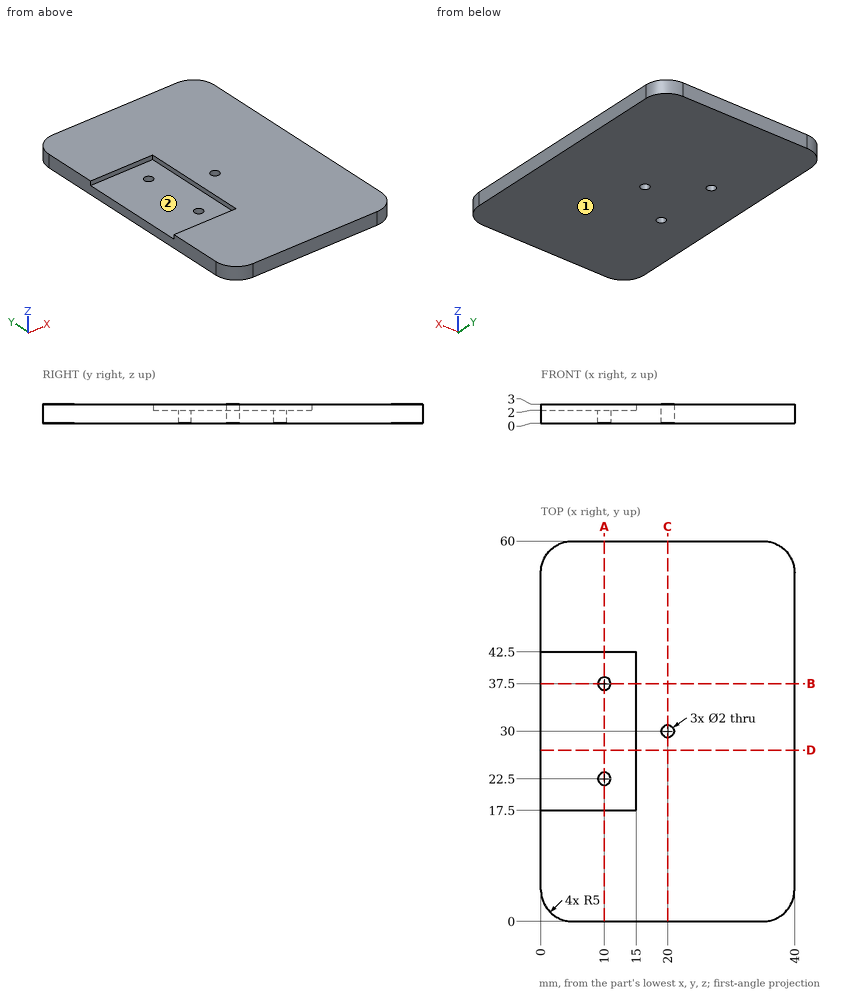
Part print with two shaded views. Sizes in mm from the minimum x, y, z corner. Coordinates: 2 decimals unless noted, no trailing zeros. Order: outer loops, then holes, each group sorted by start corner. A loop starts at its lowest first (then second) coordinate and runs counter-clockwise, first axis right, second up.
(1) Saw through at A-A, the plane x = 10. Write the cut outline in (y, z), and give its area (3 significant figures).
Solution:
outline: (0, 0) - (21.5, 0) - (21.5, 2) - (17.5, 2) - (17.5, 3) - (0, 3) - close; (23.5, 0) - (36.5, 0) - (36.5, 2) - (23.5, 2) - close; (38.5, 0) - (60, 0) - (60, 3) - (42.5, 3) - (42.5, 2) - (38.5, 2) - close
area: 147 mm2
(2) Pin check, flat tips, straight feed: pin 1 Ø2.5 at (x, y) = (10, 37.5) entering from +Z; pin 2 Ø0.5 at (y, z) = (34, 2.5) entering from -X. Stop position of each tip, or through.
Solution:
pin 1: stops at z = 2
pin 2: stops at x = 15
(3) Drill centre lines: L1, parallel to Y at x = 10, z = 0.9; L2, parallel to Y at x = 20, z = 1.6; L3, parallel to X at y = 33.5, z = 2.75. Where is each one in solid material? Low to high.
Solution:
L1: y = 0 to 21.5, 23.5 to 36.5, 38.5 to 60
L2: y = 0 to 29, 31 to 60
L3: x = 15 to 40
(4) Saw through at D-D, the plane y = 27. Write the cut outline in (x, z).
Solution:
outline: (0, 0) - (40, 0) - (40, 3) - (15, 3) - (15, 2) - (0, 2) - close
(5) Mould opens along Y. For the marked faces 1 and 2 say: released by +Y, released by -Y, zero draft, split by the parting line, or undercut.
Solution:
face 1: zero draft
face 2: undercut
(6) Saw through at C-C, the plane x = 20. Write the cut outline in (y, z).
Solution:
outline: (0, 0) - (29, 0) - (29, 3) - (0, 3) - close; (31, 0) - (60, 0) - (60, 3) - (31, 3) - close
(7) Saw through at B-B, the plane y = 37.5. Write the cut outline in (x, z).
Solution:
outline: (0, 0) - (9, 0) - (9, 2) - (0, 2) - close; (11, 0) - (40, 0) - (40, 3) - (15, 3) - (15, 2) - (11, 2) - close
